Geometry: final body of the model. Coordinates: model frame, mm. Face numbers are marked on the shaded views. A direction names the side the tool comes from. Give positions to 0.01 mm unless a question says otherwise; leave off trailing zeros. Loops run counter-clockwise (first coordinate to the right, second up) from the corner with the lowest first, then second, coordinate; pieces in that order, holes last.
```python
from build123d import *

# Parameters (mm, degrees)
CUT_EXTRUDE1_REACH = 37.93
SKETCH3_R          = 1.5
CIRPATTERN1_COUNT  = 3


with BuildPart() as part:
    # Sketch2 → Revolve1 (revolve)
    with BuildSketch(Plane.XY, mode=Mode.PRIVATE) as revolve1_sk:
        Polygon((0, 15), (28, 15), (28, 7.5), (29, 7.5), (29, 7), (0, 7), align=None)
    revolve(revolve1_sk.sketch.rotate(Axis((0, 0, 0), (1, 0, 0)), 90), axis=Axis((0, 0, 0), (1, 0, 0)))

    # Sketch3 → Cut-Extrude1 (cut, up to next)
    with BuildSketch(Plane.ZY, mode=Mode.PRIVATE) as cut_extrude1_sk1:
        with Locations((0, 10)):
            Circle(SKETCH3_R)
    cut_extrude1_tool1 = extrude(cut_extrude1_sk1.sketch, amount=-CUT_EXTRUDE1_REACH, mode=Mode.PRIVATE) & part.part
    cut_extrude1 = cut_extrude1_tool1.solids().sort_by_distance((0, 10, 0))[0]
    add(cut_extrude1, mode=Mode.SUBTRACT)

    # CirPattern1: Cut-Extrude1 ×3 about axis
    cirpattern1_axis = Axis((0, 0, 0), (1, 0, 0))
    for i in range(1, CIRPATTERN1_COUNT):
        add(cut_extrude1.rotate(cirpattern1_axis, i * 360 / CIRPATTERN1_COUNT), mode=Mode.SUBTRACT)


solid = part.part
```
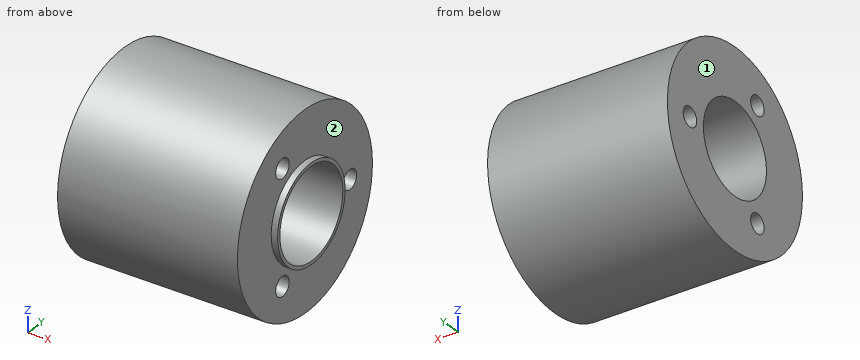
Q1. Material intervals for probe 1 along Y at (x, z) = (20, 0); probe 2 along Z at (x, y) = (18.5, 0.25); probe 3 along X at (y, z) = (-7.5, -2.75), sorted ascending.
Q2. Section query C-C, the plane y = -5. Return loops of the section in (x, z).
Q3. Section query D-D, the plane x = 23.5. Return loops of the section in (y, z), and give its area (3 significant figures).
Q4. Reachability of the marked faces 1 and 2 from +Z, -Z, +X, -X, +Y, -Y: full face, straight path, thin tool, end or side. Return the list, or none.
Q5. Section query B-B, the plane y = 0. Return loops of the section in (x, z).
Q6. Pin query (flat end, axial travel): pin 1 Ø3 at (x, y) = (23, -10) entering from -Z; pin 2 Ø4 at (x, z) = (26, 8) entering from -Y; pin 3 Ø3 at (y, z) = (2.5, 8.5) entering from -X; pin 4 Ø1.5 at (x, z) = (8.5, -1) entering from -Y. Return the tip coordinate at first contact, or that it passes through.
Q7. Section query A-A, the plane z = 0. Return loops of the section in (x, y), and give its area (3 significant figures).
Resolved:
1. probe 1: y = -15 to -7, 7 to 8.5, 11.5 to 15
1. probe 2: z = -15 to -7, 7 to 15
1. probe 3: x = 0 to 28
2. outline: (0, -14.14) - (28, -14.14) - (28, -10.16) - (0, -10.16) - close; (0, -7.16) - (28, -7.16) - (28, -5.59) - (29, -5.59) - (29, -4.9) - (0, -4.9) - close; (0, 4.9) - (29, 4.9) - (29, 5.59) - (28, 5.59) - (28, 7.16) - (0, 7.16) - close; (0, 10.16) - (28, 10.16) - (28, 14.14) - (0, 14.14) - close
3. outline: circle Ø30 at (0, 0); hole circle Ø14 at (0, 0); hole circle Ø3 at (-5, -8.66); hole circle Ø3 at (-5, 8.66); hole circle Ø3 at (10, 0)
3. area: 532 mm2
4. face 1: +Z, -Z, -X, +Y, -Y
4. face 2: +X
5. outline: (0, -15) - (28, -15) - (28, -7.5) - (29, -7.5) - (29, -7) - (0, -7) - close; (0, 7) - (29, 7) - (29, 7.5) - (28, 7.5) - (28, 15) - (0, 15) - close
6. pin 1: stops at z = -12.36
6. pin 2: stops at y = -13.75
6. pin 3: stops at x = 0
6. pin 4: stops at y = -15
7. outline: (0, -15) - (28, -15) - (28, -7.5) - (29, -7.5) - (29, -7) - (0, -7) - close; (0, 7) - (29, 7) - (29, 7.5) - (28, 7.5) - (28, 8.5) - (0, 8.5) - close; (0, 11.5) - (28, 11.5) - (28, 15) - (0, 15) - close
7. area: 365 mm2
